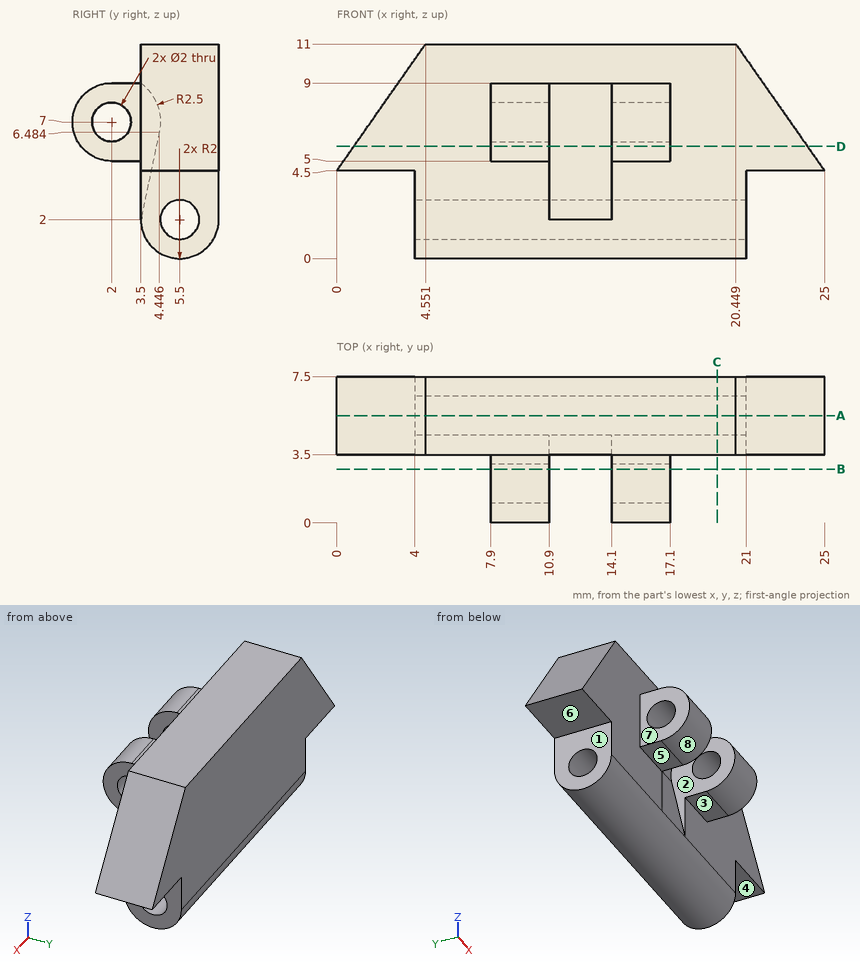
Geometry check sheet. Reference: drawing and pictorial views, mm from the part's lowest x, y, z. A direction names the side the tool comes from. Round coordinates to 2 decimals unless told otherwise and drop trailing zeros. Write each loop counter-clockwise with the first axis right and the second up, starting at its lowest first coordinate (ties: lowest second). Pieces come first, ordered by that corner, then holes. Notation, with made-up numbers: (-7, 42) -> (3, 42) arc R11 ccw to (3, 53) -> close; hole circle Ø2 at (-35.75, 35.25). An arc over 180 degrees is marked (long way). Answer as CSV lines item,"result". Start each with the question number.
1) Section check C-C on x = 19.5. Enter the section's corners in (y, z).
2) Material ranges on line 1 (Z direction, x = 16, y = 2); line 2 (Y direction, x = 14, z = 2); line 3 (Y direction, x = 8.7, z = 7), recorded low to high. Write a range as from..to.
3) Section check A-A on y = 5.5. Enter the section's corners in (x, z).
4) Go/stop test with flat-tipped pins: P1, Ø1.2, axis at x = 2, y = 6.5, coming from the -Z side; P2, Ø3, axis at x = 9, z = 1, coming from the -Y side; P3, Ø1, axis at x = 2.5, y = 3.5, coming from the +Z side (1 decimal); P4, Ø2.5, axis at y = 2.5, z = 4.5, coming from the +X side. Record where each tip stops, or that it passes through.
5) Tool access check on the marked faces 4, 5, 6, 7 and 8. Record the directions out of +Z, -Z, +X, -X, +Y, -Y that give a thin tool (end or side, any length) a straight path to the whole face; none if there is none.
6) Release check for a two-part mould opening along X. For the marked faces 1, 2 and 3 record: pulls with the +X half, pulls with the -X half, needs draft (parallel to the pull), parting line crosses it, or undercut.
7) Section check B-B on y = 2.75. Enter the section's corners in (x, z).
8) Section check D-D on z = 5.75. Enter the section's corners in (x, y) (1 decimal), and give its area (3 significant figures).
Found:
1,outline,"(3.5, 2) arc R2 ccw to (7.5, 2) -> (7.5, 11) -> (3.5, 11) -> close; hole circle Ø2 at (5.5, 2)"
2,line 1,"z = 5..6, 8..9"
2,line 2,"y = 3.5..4.5, 6.5..7.5"
2,line 3,"y = 0..1, 3..7.5"
3,outline,"(0, 4.5) -> (4, 4.5) -> (4, 3) -> (21, 3) -> (21, 4.5) -> (25, 4.5) -> (20.45, 11) -> (4.55, 11) -> close; (4, 0) -> (21, 0) -> (21, 1) -> (4, 1) -> close"
4,P1,"stops at z = 4.5"
4,P2,"stops at y = 3.5"
4,P3,"stops at z = 8.8"
4,P4,"stops at x = 25"
5,face 4,"-Z, +X, +Y, -Y"
5,face 5,"-Z, +X, -X, -Y"
5,face 6,"-Z, -X, +Y, -Y"
5,face 7,"+Z, -Z, -X, -Y"
5,face 8,"+X, -X, -Y"
6,face 1,"pulls with the -X half"
6,face 2,"undercut"
6,face 3,"needs draft"
7,outline,"(7.9, 5) -> (10.9, 5) -> (10.9, 6.34) -> (7.9, 6.34) -> close; (7.9, 7.66) -> (10.9, 7.66) -> (10.9, 9) -> (7.9, 9) -> close; (14.1, 5) -> (17.1, 5) -> (17.1, 6.34) -> (14.1, 6.34) -> close; (14.1, 7.66) -> (17.1, 7.66) -> (17.1, 9) -> (14.1, 9) -> close"
8,outline,"(0.9, 3.5) -> (7.9, 3.5) -> (7.9, 0.4) -> (10.9, 0.4) -> (10.9, 4.3) -> (14.1, 4.3) -> (14.1, 0.4) -> (17.1, 0.4) -> (17.1, 3.5) -> (24.1, 3.5) -> (24.1, 7.5) -> (0.9, 7.5) -> close"
8,area,"109 mm^2"
